```python
from build123d import *

# Parameters (mm, degrees)
F0_W       = 65
F0_H       = 46
F1_DEPTH   = 65
F2_W       = 35
F2_H       = 16
F3_DEPTH   = 45
F4_R       = 2
F5_W       = 75
F5_H       = 53.7899285555
F6_DEPTH   = 150
F7_W       = 40
F7_H       = 21
F8_DEPTH   = 110
F9_R       = 2
F10_R      = 2
F11_R      = 2
F12_W      = 150.7326364517
F12_H      = 343.7213376164
F6_FACE1_W = 75
F6_FACE1_H = 150
F1_FACE1_W = 65
F1_FACE1_H = 65
F13_DEPTH  = 26.8959642777
F14_R      = 7.75
F14_R_2    = 5.25
F15_DEPTH  = 6
F15_TAPER  = 10
F16_W      = 143.152281642
F16_H      = 267.6325216889
F17_DEPTH  = 10


with BuildPart() as f1:
    # F0 (on Top) → F1 (new body)
    with BuildSketch(Plane.XY):
        Rectangle(F0_W, F0_H)
    extrude(amount=F1_DEPTH)

    # F2 (on face) → F3 (cut)
    with BuildSketch(Plane.XY.offset(65)):
        Rectangle(F2_W, F2_H)
    extrude(amount=-F3_DEPTH, mode=Mode.SUBTRACT)

    # F4
    f4_edges = [f1.edges().sort_by_distance(p)[0] for p in [
        (-17.5, -8, 42.5),
        (-17.5, 8, 42.5),
        (17.5, -8, 42.5),
        (17.5, 8, 42.5),
    ]]
    fillet(f4_edges, radius=F4_R)

    # F5 (on face) → F6 (join)
    with BuildSketch(Plane.XY.offset(65)):
        Rectangle(F5_W, F5_H)
    extrude(amount=F6_DEPTH)

    # F7 (on face) → F8 (cut)
    with BuildSketch(Plane(origin=(0, 0, 65), x_dir=(1, 0, 0), z_dir=(0, 0, -1))):
        Rectangle(F7_W, F7_H)
    extrude(amount=-F8_DEPTH, mode=Mode.SUBTRACT)

    # F9
    f9_edges = [f1.edges().sort_by_distance(p)[0] for p in [
        (-20, -10.5, 120),
    ]]
    fillet(f9_edges, radius=F9_R)

    # F10
    f10_edges = [f1.edges().sort_by_distance(p)[0] for p in [
        (-20, 10.5, 120),
    ]]
    fillet(f10_edges, radius=F10_R)

    # F11
    f11_edges = [f1.edges().sort_by_distance(p)[0] for p in [
        (20, -10.5, 120),
        (20, 10.5, 120),
    ]]
    fillet(f11_edges, radius=F11_R)

    # F12 (on Front) + F6_face1 (on face) + F1_face1 (on face) → F13 (cut, through all)
    with BuildSketch(Plane.XZ):
        with Locations((0, 126.5255063772)):
            Rectangle(F12_W, F12_H)
    with BuildSketch(Plane(origin=(0, -26.8949642777, 140), x_dir=(1, 0, 0), z_dir=(0, -1, 0))):
        Rectangle(F6_FACE1_W, F6_FACE1_H)
    with BuildSketch(Plane(origin=(0, -23, 32.5), x_dir=(1, 0, 0), z_dir=(0, -1, 0))):
        Rectangle(F1_FACE1_W, F1_FACE1_H)
    extrude(amount=F13_DEPTH, mode=Mode.SUBTRACT)

    # F14 (on face) → F15 (cut)
    with BuildSketch(Plane.XZ):
        with Locations((0, 200)):
            Circle(F14_R)
        with Locations((0, 10)):
            Circle(F14_R_2)
    extrude(amount=-F15_DEPTH, taper=F15_TAPER, mode=Mode.SUBTRACT)

    # F16 (on face) → F17 (cut)
    with BuildSketch(Plane(origin=(0, 26.8949642777, 0), x_dir=(-1, 0, 0), z_dir=(0, 1, 0))):
        with Locations((18.2788968086, 90.5453972518)):
            Rectangle(F16_W, F16_H)
    extrude(amount=-F17_DEPTH, mode=Mode.SUBTRACT)


solid = f1.part
```
For this review, take the finished solid that the model builds, in its own axes (mm). A direction names the side the tool comes from. Round coordinates to 2 decimals unless told otherwise and drop trailing zeros. Order: outer loops, then holes, each group sorted by start corner. A loop starts at its lowest first (then second) coordinate and runs counter-clockwise, first axis right, second up.
Q1. We need section A-A, the plane y = 15. Give the boundary of the cut face in (x, z), plus the area to 3 significant figures.
Findings below:
outline: (-37.5, 65) - (-32.5, 65) - (-32.5, 0) - (32.5, 0) - (32.5, 65) - (37.5, 65) - (37.5, 215) - (-37.5, 215) - close
area: 15,500 mm2
Q2. Insertion check: P1, Ø6.5, axis at y = 4, z = 31.5, coming from the +X side; P2, Ø6, axis at x = 7, z = 39.5, coming from the -Y side; P3, Ø2.5, axis at x = 36, y = 7, coming from the -Z side. Each pin has a flat end and moves straight along its axis. Give the tip position at first contact, or say it passes through.
Findings below:
P1: stops at x = 32.5
P2: stops at y = 8
P3: stops at z = 65
Q3. Wall thickness on line 1 (Z direction, x = -13.5, y = 9.25); line 2 (X direction, y = 2, z = 117.5); line 3 (Z direction, x = 6, y = 4.25): over which ranges is each line inside the solid? List them lowest first.
Findings below:
line 1: z = 0 to 65, 175 to 215
line 2: x = -37.5 to -20, 20 to 37.5
line 3: z = 0 to 20, 175 to 196.39, 203.61 to 215
Q4. Mouldability with a two-part tool opening along Y and no side actions: class faces 5 (the conical face through (3.752, 4.375, 205.884)), 6 (the flat face through (1, 16.895, 109)), 7 (the flat face through (-1, 9, 215)) as pulls with the +Y half, pulls with the -Y half, needs draft (parallel to the pull), parting line crosses it, or undercut.
Findings below:
face 5: pulls with the -Y half
face 6: pulls with the +Y half
face 7: needs draft
Q5. We need section B-B, the plane x = 13.5. Give the boundary of the cut face in (y, z).
Findings below:
outline: (0, 0) - (16.89, 0) - (16.89, 215) - (0, 215) - (0, 175) - (10.5, 175) - (10.5, 65) - (8, 65) - (8, 20) - (0, 20) - close
Q6. We need section C-C, the plane z = 76. Give the boundary of the cut face in (x, y), plus the area to 3 significant figures.
Findings below:
outline: (-37.5, 0) - (-20, 0) - (-20, 8.5) arc R2 cw to (-18, 10.5) - (18, 10.5) arc R2 cw to (20, 8.5) - (20, 0) - (37.5, 0) - (37.5, 16.89) - (-37.5, 16.89) - close
area: 849 mm2
Q7. We need section D-D, the plane x = 0. Give the boundary of the cut face in (y, z), plus the area to 3 significant figures.
Findings below:
outline: (0, 0) - (16.89, 0) - (16.89, 215) - (0, 215) - (0, 207.75) - (6, 206.69) - (6, 193.31) - (0, 192.25) - (0, 175) - (10.5, 175) - (10.5, 65) - (8, 65) - (8, 20) - (0, 20) - (0, 15.25) - (6, 14.19) - (6, 5.81) - (0, 4.75) - close
area: 1,970 mm2
Q8. Machinability: for faces 1 (the flat face through (0, 6, 200)), 2 (the flat face through (-35, 9, 65)), 3 (the flat face through (37.5, 8, 139)), 4 (the flat face through (35, 9, 65)), which of the approach directions +Z, -Z, +X, -X, +Y, -Y give a long, thin tool a straight path to every point of the face, cutting with its end or side? Answer none if there is none.
Findings below:
face 1: -Y
face 2: -Z, -X, +Y, -Y
face 3: +Z, -Z, +X, +Y, -Y
face 4: -Z, +X, +Y, -Y
